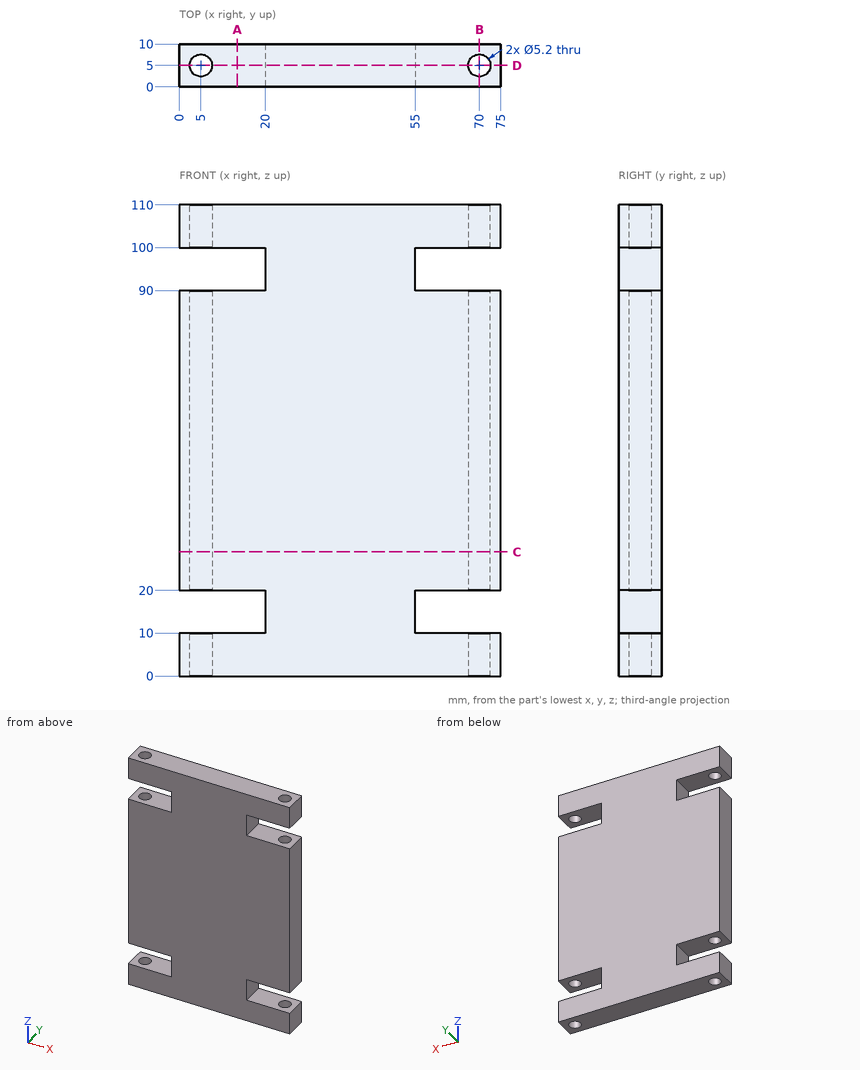
For this review, use the dimensioned drawing (mm, ordinates from the lowest corner) and the shaded views. Coordinates: 2 decimals unless noted, no trailing zeros. Order: outer loops, then holes, each group sorted by start corner. A loop starts at its lowest first (then second) coordinate and runs counter-clockwise, first axis right, second up. Notation, with made-up numbers: (10.25, -10) - (35.25, -10) arc R35 cw to (35.25, 22) - close; hole circle Ø11 at (70, 16.5). An arc over 180 degrees is marked (long way). Answer as a JSON object with one key per item and string values. Group by question number.
1. We need section B-B on x = 70. State the section outline as (y, z) points, then the cut area to 3 significant figures.
2. We need section D-D on y = 5. Give the number of separate pieces and of enclosed holes in the cut face, then the cut area to 3 significant figures.
3. Clearance check with flat-ended pins moving along their axes: P1, Ø3, axis at x = 5, y = 5, coming from the +Z side; P2, Ø5, axis at y = 3, z = 13.5, coming from the -X side. State where each tip first meets the part, or that it passes through.
4. For probe 1 along Z at (x, y) = (60, 2.75); probe 2 along Y at (x, z) = (5, 2); probe 3 along X at (y, z) = (6.5, 55.5), list the stretches that pass through material, from the lowest coordinate up.
5. We need section C-C on z = 29. State the section outline as (x, y) points, then the cut area to 3 significant figures.
6. We need section A-A on x = 13.5. State the section outline as (y, z) points.
Final values:
{
 "1": {"outline": "(0, 0) - (2.4, 0) - (2.4, 10) - (0, 10) - close; (0, 20) - (2.4, 20) - (2.4, 90) - (0, 90) - close; (0, 100) - (2.4, 100) - (2.4, 110) - (0, 110) - close; (7.6, 0) - (10, 0) - (10, 10) - (7.6, 10) - close; (7.6, 20) - (10, 20) - (10, 90) - (7.6, 90) - close; (7.6, 100) - (10, 100) - (10, 110) - (7.6, 110) - close", "area": "432 mm²"},
 "2": {"separate pieces": "7", "enclosed holes": "0", "area": "6,510 mm²"},
 "3": {"P1": "through", "P2": "x = 20"},
 "4": {"probe 1": "0 to 10, 20 to 90, 100 to 110", "probe 2": "0 to 2.4, 7.6 to 10", "probe 3": "0 to 2.88, 7.12 to 67.88, 72.12 to 75"},
 "5": {"outline": "(0, 0) - (75, 0) - (75, 10) - (0, 10) - close; hole circle Ø5.2 at (5, 5); hole circle Ø5.2 at (70, 5)", "area": "708 mm²"},
 "6": {"outline": "(0, 0) - (10, 0) - (10, 10) - (0, 10) - close; (0, 20) - (10, 20) - (10, 90) - (0, 90) - close; (0, 100) - (10, 100) - (10, 110) - (0, 110) - close"}
}
